Input: part model. Units: mm. Frame: model coordinates. Coordinates: 2 decimals unless noted, no trailing zeros. Loops run counter-clockwise (first coordinate to the right, second up) from the corner with the lowest first, then second, coordinate; pieces in that order, holes last. Notation, with made-up numbers: M 77,-38.5 L 125,-38.5 A16 cw 125,-15.5 Z; hole C 62,15 d6. An arc over 180 degrees is marked long. Use a Markdown table: item, result. Add a question column.
1. Section B-B on x = 7.5. Output: boundary loops of the cut face in (y, z).
2. Section A-A on x = 1.25. Output: boundary loops of the cut face in (y, z), then the cut area to 3 significant figures.
3. Draft query along Z for faces 1 (the flat face through (2, 2.6, -1.5)), 2 (the cylindrical face through (10, 2, 0)). Return one class per face: +Z half, -Z half, draft (parallel to the pull), parting line (faces both ways), or undercut.
4. Line query: L1, parallel to Y at x = 2.75, z = -2.75; L2, parallel to Z at x = 2.25, y = -2; L3, parallel to X at y = 0.25, z = 0.5. Output: solid intervals per line, ascending. Write a range as [from, to].
5. Pin query (flat end, axial travel): pin 1 (2 mm diameter, centred on x = 9.5, y = 1.5, fed in from +Z); pin 2 (1.2 mm diameter, centred on y = 1.5, z = 2, fed in from -X). Return the tip coordinate at first contact, or that it passes through.
```python
from build123d import *

# Parameters (mm, degrees)
CHAMFER1_SIZE      = 0.625
CUT_EXTRUDE1_DEPTH = 4
CHAMFER2_SIZE      = 0.8
FILLET1_R          = 0.4


with BuildPart() as part:
    # Sketch1 → Revolve1 (revolve)
    with BuildSketch(Plane(origin=(0, 0, 0), x_dir=(1, 0, 0), z_dir=(0, 1, 0))):
        Polygon((0, 0), (0, 4), (5, 4), (5, 2), (15, 2), (15, 0), align=None)
    revolve(axis=Axis((15, 0, 0), (-1, 0, 0)))

    # Chamfer1
    chamfer1_edges = [part.edges().sort_by_distance(p)[0] for p in [
        (15, 0, 2),
    ]]
    chamfer(chamfer1_edges, length=CHAMFER1_SIZE)

    # Sketch3 → Cut-Revolve1 (revolve, cut)
    with BuildSketch(Plane(origin=(0, 0, 0), x_dir=(1, 0, 0), z_dir=(0, 1, 0)), mode=Mode.PRIVATE) as cut_revolve1_sk:
        Polygon((0, 0), (5.732050808, 0), (4, 3), (0, 3), align=None)
    revolve(cut_revolve1_sk.sketch.rotate(Axis((0, 0, 0), (1, 0, 0)), 180), axis=Axis((0, 0, 0), (1, 0, 0)), mode=Mode.SUBTRACT)

    # Sketch2 → Cut-Extrude1 (cut)
    with BuildSketch(Plane.ZY):
        Polygon((0, 3.464101615), (-3, 1.732050808), (-3, -1.732050808), (0, -3.464101615), (3, -1.732050808), (3, 1.732050808), align=None)
    extrude(amount=-CUT_EXTRUDE1_DEPTH, mode=Mode.SUBTRACT)

    # Chamfer2
    # the kernel refuses this chamfer: 0.8 mm, written as the material it takes off along each edge
    with BuildSketch(Plane(origin=(0, 0, 0), x_dir=(0, 0, -1), z_dir=(0, 1, 0))) as chamfer2_piece_1:
        Polygon((4, -CHAMFER2_SIZE), (4 - CHAMFER2_SIZE, 0), (4, 0), align=None)
    revolve(axis=Axis((0, 0, 0), (-1, 0, 0)), mode=Mode.SUBTRACT)

    # Fillet1
    fillet1_edges = [part.edges().sort_by_distance(p)[0] for p in [
        (5, 0, 2),
    ]]
    fillet(fillet1_edges, radius=FILLET1_R)


solid = part.part
```
Answers below:
| question | item | result |
|---|---|---|
| 1 | outline | C 0,0 d4 |
| 2 | outline | C 0,0 d8; hole M -3.46,0 L -1.73,-3 L 1.73,-3 L 3.46,0 L 1.73,3 L -1.73,3 Z |
| 2 | area | 19.1 mm² |
| 3 | face 1 | undercut |
| 3 | face 2 | parting line |
| 4 | L1 | y = [-2.9, -1.88], [1.88, 2.9] |
| 4 | L2 | z = [-3.46, -2.54], [2.54, 3.46] |
| 4 | L3 | x = [5.41, 15] |
| 5 | pin 1 | stops at z = 1.94 |
| 5 | pin 2 | stops at x = 4 |
